from build123d import *

# Parameters (mm, degrees)
SKETCH1_W                                     = 139.7
SKETCH1_H                                     = 139.7
PLATE_DEPTH                                   = 3.175
SKETCH2_R                                     = 5.08
FORCE_SENSOR_POST_HOLES_DEPTH                 = 99.833828343
GUIDANCE_SCREW_HOLES_10_CLEARANCE_D           = 5.1054
GEARBOX_MOUNT_HOLES_4_CLEARANCE_D             = 3.2639
GEARBOX_MOUNT_HOLES_4_CLEARANCE_DEPTH         = 7.62
GEARBOX_MOUNT_HOLES_4_CLEARANCE_TIP           = 0.980574487
BEARING_MOUNT_HOLES_4_CLEARANCE_D             = 3.2639
BEARING_MOUNT_HOLES_4_CLEARANCE_DEPTH         = 7.62
BEARING_MOUNT_HOLES_4_CLEARANCE_TIP           = 0.980574487
FORCE_SENSOR_FOUNDATION_HOLES_10_CLEARA_D     = 5.1054
FORCE_SENSOR_FOUNDATION_HOLES_10_CLEARA_DEPTH = 7.62
FORCE_SENSOR_FOUNDATION_HOLES_10_CLEARA_TIP   = 1.533816902
BALL_CASTER_MOUNT_HOLES_4_CLEARANCE_D         = 3.2639
BALL_CASTER_MOUNT_HOLES_4_CLEARANCE_DEPTH     = 7.62
BALL_CASTER_MOUNT_HOLES_4_CLEARANCE_TIP       = 0.980574487


with BuildPart() as part:
    # Sketch1 → Plate (new body)
    with BuildSketch(Plane(origin=(0, 0, 0), x_dir=(1, 0, 0), z_dir=(0, 1, 0))):
        Rectangle(SKETCH1_W, SKETCH1_H)
    extrude(amount=PLATE_DEPTH)

    # Sketch2 → Force Sensor Post Holes (cut, through all)
    with BuildSketch(Plane(origin=(0, 3.175, 0), x_dir=(1, 0, 0), z_dir=(0, 1, 0))):
        with Locations(Location((-22.225, 11.43, 0), (0, 0, 270))):
            Circle(SKETCH2_R)
        with Locations(Location((22.225, 11.43, 0), (0, 0, 270))):
            Circle(SKETCH2_R)
    extrude(amount=-FORCE_SENSOR_POST_HOLES_DEPTH, mode=Mode.SUBTRACT)

    # Guidance Screw Holes (#10 clearance) (through all)
    with Locations(Plane(origin=(0, 3.175, 0), x_dir=(1, 0, 0), z_dir=(0, 1, 0))):
        with Locations((63.5, -63.5), (-60.325, 19.05), (63.5, 60.325)):
            Hole(GUIDANCE_SCREW_HOLES_10_CLEARANCE_D / 2)

    # Gearbox Mount Holes (#4 clearance)
    with Locations(Plane(origin=(0, 3.175, 0), x_dir=(1, 0, 0), z_dir=(0, 1, 0))):
        with Locations((-60.96, -51.562), (-42.545, -42.037), (-24.13, -51.562), (-42.545, -61.087)):
            Hole(GEARBOX_MOUNT_HOLES_4_CLEARANCE_D / 2, depth=GEARBOX_MOUNT_HOLES_4_CLEARANCE_DEPTH)
            with Locations((0, 0, -(GEARBOX_MOUNT_HOLES_4_CLEARANCE_DEPTH + GEARBOX_MOUNT_HOLES_4_CLEARANCE_TIP / 2))):  # 118° drill point
                Cone(0, GEARBOX_MOUNT_HOLES_4_CLEARANCE_D / 2, GEARBOX_MOUNT_HOLES_4_CLEARANCE_TIP, mode=Mode.SUBTRACT)

    # Bearing Mount Holes (#4 clearance)
    with Locations(Plane(origin=(0, 3.175, 0), x_dir=(1, 0, 0), z_dir=(0, 1, 0))):
        with Locations((25.0825, -38.0365), (51.6509, -38.0365), (25.0825, -65.0875), (51.6509, -65.0875)):
            Hole(BEARING_MOUNT_HOLES_4_CLEARANCE_D / 2, depth=BEARING_MOUNT_HOLES_4_CLEARANCE_DEPTH)
            with Locations((0, 0, -(BEARING_MOUNT_HOLES_4_CLEARANCE_DEPTH + BEARING_MOUNT_HOLES_4_CLEARANCE_TIP / 2))):  # 118° drill point
                Cone(0, BEARING_MOUNT_HOLES_4_CLEARANCE_D / 2, BEARING_MOUNT_HOLES_4_CLEARANCE_TIP, mode=Mode.SUBTRACT)

    # Force Sensor Foundation Holes (#10 clearance)
    with Locations(Plane(origin=(0, 3.175, 0), x_dir=(1, 0, 0), z_dir=(0, 1, 0))):
        with Locations((-36.6395, 22.5425), (36.3855, 22.5425), (36.3855, 0.3175), (-36.6395, 0.3175), (0, 0.3175), (0, 22.5425)):
            Hole(FORCE_SENSOR_FOUNDATION_HOLES_10_CLEARA_D / 2, depth=FORCE_SENSOR_FOUNDATION_HOLES_10_CLEARA_DEPTH)
            with Locations((0, 0, -(FORCE_SENSOR_FOUNDATION_HOLES_10_CLEARA_DEPTH + FORCE_SENSOR_FOUNDATION_HOLES_10_CLEARA_TIP / 2))):  # 118° drill point
                Cone(0, FORCE_SENSOR_FOUNDATION_HOLES_10_CLEARA_D / 2, FORCE_SENSOR_FOUNDATION_HOLES_10_CLEARA_TIP, mode=Mode.SUBTRACT)

    # Ball Caster Mount Holes (#4 clearance)
    with Locations(Plane(origin=(0, 3.175, 0), x_dir=(1, 0, 0), z_dir=(0, 1, 0))):
        with Locations((-35.306, 57.531), (-54.229, 57.531), (-54.229, 38.608), (-54.229, 2.794), (-54.229, -16.129), (-35.306, -16.129), (35.306, -16.129), (54.229, -16.129), (54.229, 2.794)):
            Hole(BALL_CASTER_MOUNT_HOLES_4_CLEARANCE_D / 2, depth=BALL_CASTER_MOUNT_HOLES_4_CLEARANCE_DEPTH)
            with Locations((0, 0, -(BALL_CASTER_MOUNT_HOLES_4_CLEARANCE_DEPTH + BALL_CASTER_MOUNT_HOLES_4_CLEARANCE_TIP / 2))):  # 118° drill point
                Cone(0, BALL_CASTER_MOUNT_HOLES_4_CLEARANCE_D / 2, BALL_CASTER_MOUNT_HOLES_4_CLEARANCE_TIP, mode=Mode.SUBTRACT)


solid = part.part
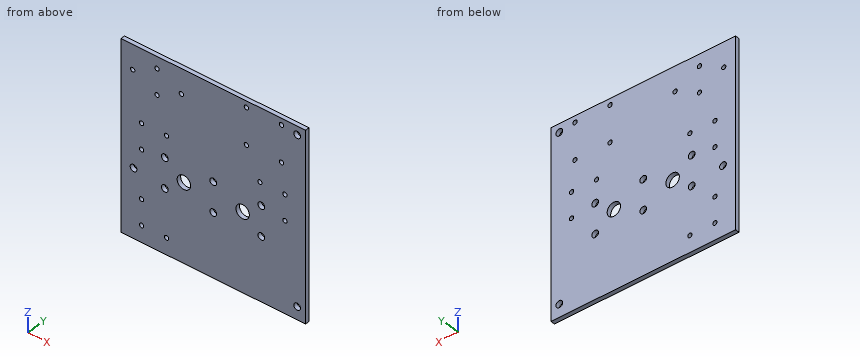
The model under review builds one solid part; all positions refer to its coordinate system, in mm. Give positions to 0.01 mm unless a question says otherwise; leave off trailing zeros. Order: outer loops, then holes, each group sorted by start corner. A loop starts at its lowest first (then second) coordinate and runs counter-clockwise, first axis right, second up. Notation, with made-up numbers: M 79.5,-16.75 L 106.5,-16.75 A6 cw 106.5,-9.75 Z; hole C 29,-9 d7. An arc over 180 degrees is marked long. Answer in a Markdown table with one row per item. Add a question column.
1. To check wall thickness, follow line 1 along X through (y, z) = (1.15, -11.43) (3 decimals); line 2 along X through (y, z) = (1.3, 1); line 3 along X through (y, z) = (1.4, 0). State the ranges of each line that lie inside material, in increasing order.
2. Add section B-B on x = -60.96. State the section outline as (y, z) points (3 decimals), plus the area to 3 significant figures.
3. Add section A-A on x = 0. State the section outline as (y, z) points (3 decimals), plus the area to 3 significant figures.
4. For pin 1 Ø2.5 at (x, z) = (51.65, 65.09) entering from +Y, flat-tipped, find the tip position at first contact; note if it passes through.
The answers:
| question | item | result |
|---|---|---|
| 1 | line 1 | -69.85 to -27.305, -17.145 to 17.145, 27.305 to 69.85 |
| 1 | line 2 | -69.85 to -38.83, -34.45 to -2.19, 2.19 to 34.2, 38.57 to 69.85 |
| 1 | line 3 | -69.85 to -39.17, -34.11 to -2.53, 2.53 to 33.85, 38.92 to 69.85 |
| 2 | outline | M 0,-69.85 L 3.175,-69.85 L 3.175,-21.522 L 0,-21.522 Z; M 0,-16.578 L 3.175,-16.578 L 3.175,49.93 L 0,49.93 Z; M 0,53.194 L 3.175,53.194 L 3.175,69.85 L 0,69.85 Z |
| 2 | area | 417 mm2 |
| 3 | outline | M 0,-69.85 L 3.175,-69.85 L 3.175,-25.095 L 0,-25.095 Z; M 0,-19.99 L 3.175,-19.99 L 3.175,-2.87 L 0,-2.87 Z; M 0,2.235 L 3.175,2.235 L 3.175,69.85 L 0,69.85 Z |
| 3 | area | 411 mm2 |
| 4 | pin 1 | through |
